Geometry: final body of the model. Coordinates: model frame, mm. Give positions to 0.01 mm unless a question says otherwise; leave off trailing zeros. Loops run counter-clockwise (first coordinate to the right, second up) from the corner with the lowest first, then second, coordinate; pieces in that order, holes last.
Autodesk Inventor part; units mm, degrees
ref_plane "YZ Plane" through (0, 0, 0) normal (1, 0, 0) x (0, 1, 0)
ref_plane "XZ Plane" through (0, 0, 0) normal (0, 1, 0) x (-1, 0, 0)
ref_plane "XY Plane" through (0, 0, 0) normal (0, 0, 1) x (1, 0, 0)
ref_plane "作業平面1" through (0, 0, 0) normal (0, 0, 1) x (1, 0, 0)
sketch "スケッチ1" plane through (0, 0, 0) normal (0, 0, 1) x (1, 0, 0)
  circle A0 centre (-6, -21.7) radius 1.25
  circle A1 centre (-19, -21.7) radius 1.25
  circle A2 centre (-19, -2.3) radius 1.25
  circle A3 centre (-6, -2.3) radius 1.25
  line L0 (0, -24) -> (-27.3, -24)
  line L1 (-3.7, -24) -> (-3.7, 4)
  line L2 (-3.7, 4) -> (-21.3, 4)
  line L3 (-21.3, 4) -> (-21.3, -24)
  circle A4 centre (-6, -21.7) radius 2.3 construction
  circle A5 centre (-19, -21.7) radius 2.3 construction
  point P0 (0, 0)
  dimension "d0" = 28
extrude "押し出し1" add sketch "スケッチ1" along normal blind 3
properties part number "KickerMount_R"
Q1. Section query C-C, the plane z = 1.15. Return loops of the section in (x, y).
Q2. Pin query (flat end, axial travel): pin 1 Ø3 at (x, y) = (-19, -2.3) entering from -Z; pin 2 Ø1.5 at (x, y) = (-6, -2.3) entering from +Z. Return the tip coordinate at first contact, or that it passes through.
Q3. Section query B-B, the plane y = -21.7. Return loops of the section in (x, z), and give its area (3 significant figures).
Q4. Material intervals for probe 1 along Y at (x, z) = (-6, 2.2); probe 2 along X at (y, z) = (-22.25, 2.85); probe 3 along Y at (x, z) = (-5.25, 0.85), sorted ascending.
Q5. Section query A-A, the plane x = -6. Return loops of the section in (y, z).
Q6. Mould query, pull axis X, two halves, no side actions, for faces 1 (the face through (-21.3, -10, 1)), 2 (the face through (-6.921, -22.545, 1.479)), 3 (the face through (-3.7, -10, 1)). Classes: +X half, -X half, draft (parallel to the pull), parting line (faces both ways), or undercut.
Resolved:
1. outline: (-21.3, -24) - (-3.7, -24) - (-3.7, 4) - (-21.3, 4) - close; hole circle Ø2.5 at (-19, -21.7); hole circle Ø2.5 at (-19, -2.3); hole circle Ø2.5 at (-6, -21.7); hole circle Ø2.5 at (-6, -2.3)
2. pin 1: stops at z = 0
2. pin 2: passes through
3. outline: (-21.3, 0) - (-20.25, 0) - (-20.25, 3) - (-21.3, 3) - close; (-17.75, 0) - (-7.25, 0) - (-7.25, 3) - (-17.75, 3) - close; (-4.75, 0) - (-3.7, 0) - (-3.7, 3) - (-4.75, 3) - close
3. area: 37.8 mm2
4. probe 1: y = -24 to -22.95, -20.45 to -3.55, -1.05 to 4
4. probe 2: x = -21.3 to -20.12, -17.88 to -7.12, -4.88 to -3.7
4. probe 3: y = -24 to -22.7, -20.7 to -3.3, -1.3 to 4
5. outline: (-24, 0) - (-22.95, 0) - (-22.95, 3) - (-24, 3) - close; (-20.45, 0) - (-3.55, 0) - (-3.55, 3) - (-20.45, 3) - close; (-1.05, 0) - (4, 0) - (4, 3) - (-1.05, 3) - close
6. face 1: -X half
6. face 2: undercut
6. face 3: +X half
